Geometry check sheet. Reference: the model listing, model coordinates, mm. Round coordinates to 2 decimals unless told otherwise and drop trailing zeros. Write each loop counter-clockwise with the first axis right and the second up, starting at its lowest first coordinate (ties: lowest second). Pieces come first, ordered by that corner, then holes. Notation, with made-up numbers: (15, -31.5) -> (56, -31.5) arc R19 ccw to (56, 1.5) -> close; hole circle Ø5 at (35.5, -3.5). An arc over 180 degrees is marked (long way). Use a Markdown table: item, result.
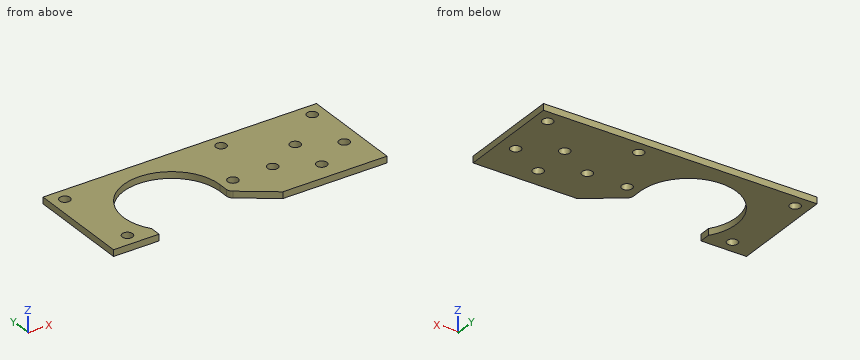
```python
from build123d import *

# Parameters (mm, degrees)
SKETCH1_R           = 2.5527
BOSS_EXTRUDE1_DEPTH = 3.175
SKETCH3_R           = 2.5527
CUT_EXTRUDE2_DEPTH  = 143.733819135
FILLET1_R           = 3.175


with BuildPart() as part:
    # Sketch1 → Boss-Extrude1 (new body)
    with BuildSketch(Plane.XY):
        with BuildLine():
            Line((0, 0), (0, 50.8))
            Line((0, 50.8), (-133.35, 50.8))
            Line((-133.35, 50.8), (-133.35, 0))
            Line((-133.35, 0), (-111.125, 0))
            Line((-111.125, 0), (-111.125, 5.298181029))
            ThreePointArc((-111.125, 5.298181029), (-99.30117724, 41.406148763), (-68.58, 19.05))
            Line((-68.58, 19.05), (-68.58, 12.7))
            Line((-68.58, 12.7), (-50.8, 0))
            Line((-50.8, 0), (0, 0))
        make_face()
        with Locations((-25.4, 9.525)):
            Circle(SKETCH1_R, mode=Mode.SUBTRACT)
        with Locations((-25.4, 28.575)):
            Circle(SKETCH1_R, mode=Mode.SUBTRACT)
        with Locations((-7.9375, 19.05)):
            Circle(SKETCH1_R, mode=Mode.SUBTRACT)
        with Locations((-42.8625, 19.05)):
            Circle(SKETCH1_R, mode=Mode.SUBTRACT)
    extrude(amount=BOSS_EXTRUDE1_DEPTH)

    # Sketch3 → Cut-Extrude2 (cut, through all)
    with BuildSketch(Plane(origin=(0, 0, 0), x_dir=(-1, 0, 0), z_dir=(0, 0, -1))):
        with Locations((122.2375, 6.35)):
            Circle(SKETCH3_R)
        with Locations((127, 44.45)):
            Circle(SKETCH3_R)
        with Locations((6.35, 44.45)):
            Circle(SKETCH3_R)
        with Locations((50.8, 44.45)):
            Circle(SKETCH3_R)
        with Locations((62.23, 19.05)):
            Circle(SKETCH3_R)
    extrude(amount=-CUT_EXTRUDE2_DEPTH, mode=Mode.SUBTRACT)

    # Fillet1
    fillet1_edges = [part.edges().sort_by_distance(p)[0] for p in [
        (-68.58, 12.7, 1.5875),
    ]]
    fillet(fillet1_edges, radius=FILLET1_R)


solid = part.part
```
(1) Section check A-A on x = -127. Record the cut outline in (y, z) (3 decimals).
A:
| item | result |
|---|---|
| outline | (0, 0) -> (41.897, 0) -> (41.897, 3.175) -> (0, 3.175) -> close; (47.003, 0) -> (50.8, 0) -> (50.8, 3.175) -> (47.003, 3.175) -> close |
(2) Thickness scan on line 1 (Y direction, x = -25.4, z = 2.55); line 2 (X direction, y = 27, z = 1.9); line 3 (X direction, y = 43.5, z = 2.8). Record the ranges inside material, lowest first.
A:
| item | result |
|---|---|
| line 1 | y = 0 to 6.97, 12.08 to 26.02, 31.13 to 50.8 |
| line 2 | x = -133.35 to -114.18, -69.97 to -27.41, -23.39 to 0 |
| line 3 | x = -133.35 to -129.37, -124.63 to -53.17, -48.43 to -8.72, -3.98 to 0 |
(3) Gauge pin test, flat ends, axial feed: pin 1 Ø6.5 at (x, y) = (-25.4, 9.525) entering from -Z; pin 2 Ø4 at (x, y) = (-6.35, 44.45) entering from +Z. Record the tip position at first contact, or that the pin passes through.
A:
| item | result |
|---|---|
| pin 1 | stops at z = 0 |
| pin 2 | passes through |
(4) Section check B-B on y = 44.45. Record the cut outline in (x, z) (3 decimals).
A:
| item | result |
|---|---|
| outline | (-133.35, 0) -> (-129.553, 0) -> (-129.553, 3.175) -> (-133.35, 3.175) -> close; (-124.447, 0) -> (-53.353, 0) -> (-53.353, 3.175) -> (-124.447, 3.175) -> close; (-48.247, 0) -> (-8.903, 0) -> (-8.903, 3.175) -> (-48.247, 3.175) -> close; (-3.797, 0) -> (0, 0) -> (0, 3.175) -> (-3.797, 3.175) -> close |
(5) Section check C-C on z = 2.4. State how many separate pieces and enclosed holes the cut face has, plus the area to 3 significant figures.
A:
| item | result |
|---|---|
| separate pieces | 1 |
| enclosed holes | 9 |
| area | 4,760 mm2 |
(6) Section check D-D on y = 37. Record the cut outline in (x, z) (3 decimals), plus the area to 3 significant figures.
A:
| item | result |
|---|---|
| outline | (-133.35, 0) -> (-107.235, 0) -> (-107.235, 3.175) -> (-133.35, 3.175) -> close; (-76.915, 0) -> (0, 0) -> (0, 3.175) -> (-76.915, 3.175) -> close |
| area | 327 mm2 |
